from build123d import *

# Parameters (mm, degrees)
F0_W     = 180
F0_H     = 31
F1_DEPTH = 2.5
F2_W     = 31
F2_H     = 60
F3_DEPTH = 2.5


with BuildPart() as f1:
    # F0 (on Top) → F1 (new body, symmetric)
    with BuildSketch(Plane.XY):
        with Locations((-21.178086, 7.692472)):
            Rectangle(F0_W, F0_H)
    extrude(amount=F1_DEPTH, both=True)

    # F2 (on Top) → F3 (join, symmetric)
    with BuildSketch(Plane.XY):
        with Locations((-97.912037, 7.913927)):
            Rectangle(F2_W, F2_H)
    extrude(amount=F3_DEPTH, both=True)


solid = f1.part
For this review, take the finished solid that the model builds, in its own axes (mm). A direction names the side the tool comes from. Round coordinates to 2 decimals unless told otherwise and drop trailing zeros. Write each loop counter-clockwise with the first axis right and the second up, starting at its lowest first coordinate (ties: lowest second). Pieces come first, ordered by that corner, then holes. Notation, with made-up numbers: (9, 2.5) -> (57, 2.5) arc R33 cw to (57, 39.5) -> close; hole circle Ø11 at (89.25, 17). An arc over 180 degrees is marked (long way). Put each result on its own line as item: value.
Q1. Consider section A-A on z = -1.5. State the section outline as (x, y) points.
Determined:
outline: (-113.41, -22.09) -> (-82.41, -22.09) -> (-82.41, -7.81) -> (68.82, -7.81) -> (68.82, 23.19) -> (-82.41, 23.19) -> (-82.41, 37.91) -> (-113.41, 37.91) -> close
Q2. Machinability: for faces 1 (the flat face through (-8, 23.192, 0)), 2 (the flat face through (-82.412, -15, 0)), 3 (the flat face through (-113.412, 7, 0)), which of the approach directions +Z, -Z, +X, -X, +Y, -Y give a long, thin tool a straight path to every point of the face, cutting with its end or side? Answer none if there is none.
Determined:
face 1: +Z, -Z, +X, +Y
face 2: +Z, -Z, +X, -Y
face 3: +Z, -Z, -X, +Y, -Y
Q3. Consider section C-C on y = -10. State the section outline as (x, z) points, and give its area (3 significant figures).
Determined:
outline: (-113.41, -2.5) -> (-82.41, -2.5) -> (-82.41, 2.5) -> (-113.41, 2.5) -> close
area: 155 mm^2
Q4. To check wall thickness, follow L1, parallel to Y at x = 37.5, z = -1.5; L2, parallel to X at y = 24.5, z = -2. State the ranges of each line that lie inside material, in increasing order. Write a range as [from, to].
Determined:
L1: y = [-7.81, 23.19]
L2: x = [-113.41, -82.41]
Q5. Consider section B-B on x = 16. State the section outline as (y, z) points, and give its area (3 significant figures).
Determined:
outline: (-7.81, -2.5) -> (23.19, -2.5) -> (23.19, 2.5) -> (-7.81, 2.5) -> close
area: 155 mm^2
Q6. Clearance check with flat-ended pins moving along their axes: pin 1 Ø1 at (x, z) = (42.5, -2) entering from +Y; pin 2 Ø2.5 at (x, z) = (26.5, -1) entering from -Y; pin 3 Ø1.5 at (y, z) = (-16, -0.5) entering from +X. State where each tip first meets the part, or that it passes through.
Determined:
pin 1: stops at y = 23.19
pin 2: stops at y = -7.81
pin 3: stops at x = -82.41
